Source: CAD feature listing. Evaluate the final solid. Frame: model axes, mm. Face numbers are marked on the shaded views. A direction names the side the tool comes from. Give positions to 0.01 mm unless a question says otherwise; leave off trailing zeros. Loops run counter-clockwise (first coordinate to the right, second up) from the corner with the lowest first, then second, coordinate; pieces in that order, holes last.
from build123d import *

# Parameters (mm, degrees)
SKETCH_W        = 24
SKETCH_H        = 15
SKETCH_R        = 3
PAD_DEPTH       = 3
SKETCH001_W     = 3
SKETCH001_H     = 20
PAD001_DEPTH    = 20
SKETCH002_R     = 1.5
POCKET_DEPTH    = 24.001
CHAMFER_SIZE    = 7
CHAMFER001_SIZE = 1


with BuildPart() as part:
    # Sketch → Pad (new body)
    with BuildSketch(Plane.XZ):
        with Locations((12, 7.5)):
            Rectangle(SKETCH_W, SKETCH_H)
        with Locations((12, 7.5)):
            Circle(SKETCH_R, mode=Mode.SUBTRACT)
    extrude(amount=PAD_DEPTH)

    # Sketch001 (on Face7 of Pad) → Pad001 (join)
    with BuildSketch(Plane.XZ.offset(3)):
        with Locations((22.5, 10)):
            Rectangle(SKETCH001_W, SKETCH001_H)
        with Locations((1.5, 10)):
            Rectangle(SKETCH001_W, SKETCH001_H)
    extrude(amount=PAD001_DEPTH)

    # Sketch002 (on Face10 of Pad001) → Pocket (cut, through all)
    with BuildSketch(Plane(origin=(24, 0, 0), x_dir=(0, 0, 1), z_dir=(1, 0, 0))):
        with Locations((12.5, 15.5)):
            Circle(SKETCH002_R)
        Polygon((20, 23), (14.25, 0), (20, 0), align=None)
        Polygon((0, 23), (5.75, 23), (0, 0), align=None)
    extrude(amount=-POCKET_DEPTH, mode=Mode.SUBTRACT)

    # Chamfer
    chamfer_edges = [part.edges().sort_by_distance(p)[0] for p in [
        (1.5, -23, 20),
        (22.5, -23, 20),
    ]]
    chamfer(chamfer_edges, length=CHAMFER_SIZE)

    # Chamfer001
    chamfer001_edges = [part.edges().sort_by_distance(p)[0] for p in [
        (22.5, -23, 5.75),
        (1.5, -23, 5.75),
    ]]
    chamfer(chamfer001_edges, length=CHAMFER001_SIZE)


solid = part.part
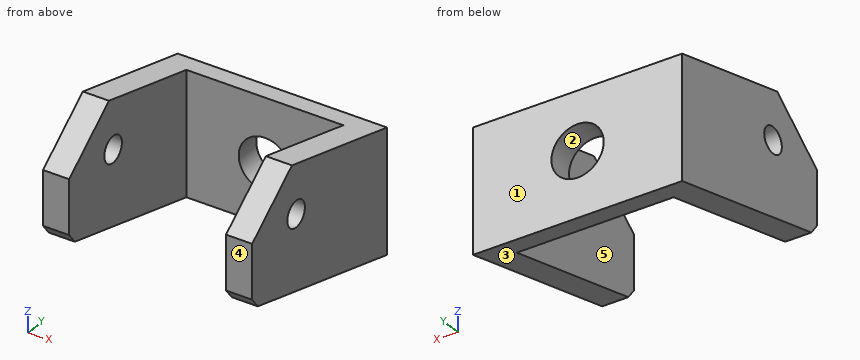
1) Pull-direction query (Z, two-part tool) for the marked faces 1, 2 and 3; classes: released by +Z, released by -Z, zero draft, split by the parting line, or undercut.
Checks:
face 1: zero draft
face 2: undercut
face 3: released by -Z
2) Cut plane A-A (x = 12). Return loops of the section in (y, z), and give its area (4 significant figures).
Checks:
outline: (-3, 0.75) - (0, 0) - (0, 4.5) - (-3, 4.5) - close; (-3, 10.5) - (0, 10.5) - (0, 14.25) - (-3, 15) - close
area: 24.75 mm2
3) Ray query, probe 1 along Y at (x, z) = (2.3, 12.5); probe 2 along X at (y, z) = (-15.25, 7.75); probe 3 along Y at (x, z) = (15.5, 2.75). Return the intervals inside material, ascending.
Checks:
probe 1: y = -23 to -17, -14 to 0
probe 2: x = 0 to 3, 21 to 24
probe 3: y = -3 to 0
4) Contact query for flat-ended pins moving along their axis: P1, Ø2, axis at x = 19.5, z = 9.5, coming from the -Y side; P2, Ø5.5, axis at x = 12, z = 7.5, coming from the -Y side. Output: stop coordinate, or through.
Checks:
P1: stops at y = -3
P2: passes through
5) Cut plane C-C (x = 22.75). Return loops of the section in (y, z), and give its area (3 significant figures).
Checks:
outline: (-23, 6.75) - (-22.03, 5.51) - (0, 0) - (0, 14.25) - (-16.21, 18.3) - (-23, 13) - close; hole circle Ø3 at (-15.5, 12.5)
area: 296 mm2
6) Cut plane B-B (z = 12.5). Return loops of the section in (x, y), and give its area (3 significant figures).
Checks:
outline: (0, -23) - (3, -23) - (3, -17) - (0, -17) - close; (0, -14) - (3, -14) - (3, -3) - (21, -3) - (21, -14) - (24, -14) - (24, 0) - (0, 0) - close; (21, -23) - (24, -23) - (24, -17) - (21, -17) - close
area: 174 mm2
7) Cut plane D-D (y = -20.25). Return loops of the section in (x, z).
Checks:
outline: (0, 5.06) - (3, 5.06) - (3, 15.15) - (0, 15.15) - close; (21, 5.06) - (24, 5.06) - (24, 15.15) - (21, 15.15) - close
8) Reachability of the marked faces 4 and 5 from +Z, -Z, +X, -X, +Y, -Y: full face, straight path, thin tool, end or side. Return the list, or none.
Checks:
face 4: +Z, -Z, +X, -X, -Y
face 5: +Z, -Z, -Y
